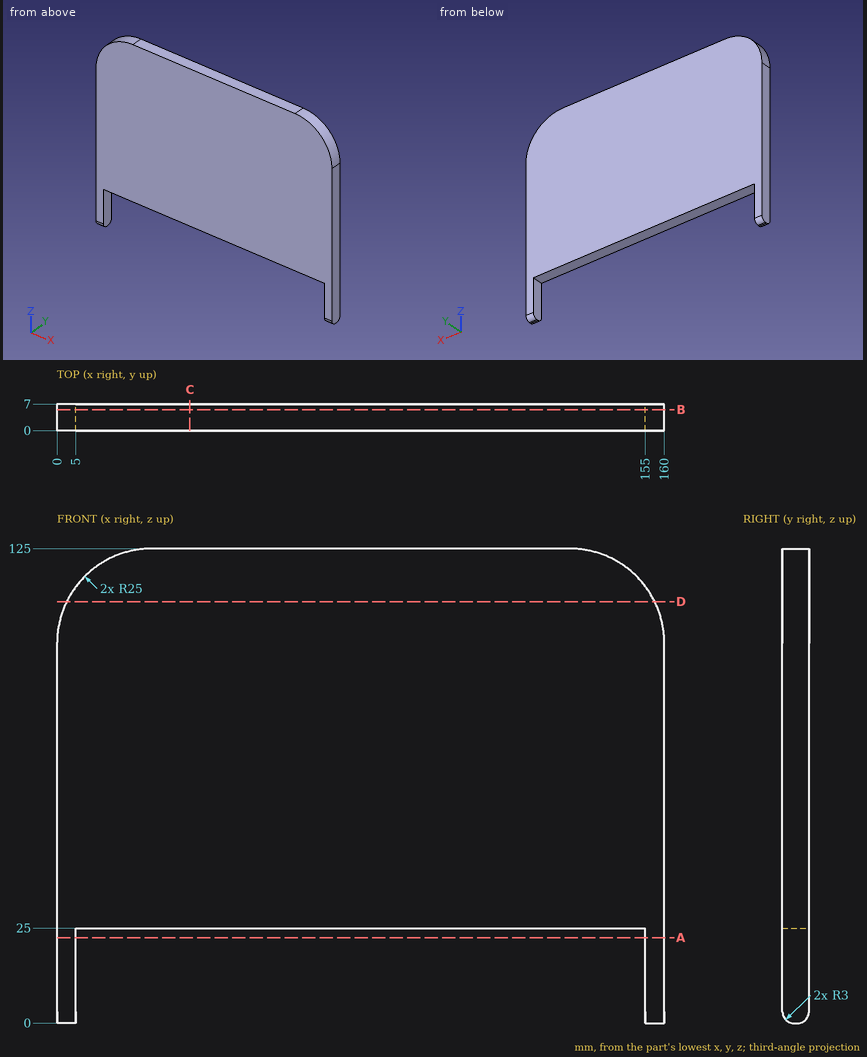
Geometry: see drawing. Coordinates: mm, zero at the bounding-box minimum. Coordinates: 2 decimals unless noted, no trailing zeros. Write each loop counter-clockwise with the first axis right and the second up, starting at its lowest first coordinate (ties: lowest second). Pieces come first, ordered by that corner, then holes. Notation, with made-up numbers: M 67,89 L 77,89 A24 ccw 77,115 Z; hole C 7.5,-13 d3. An arc over 180 degrees is marked long. Answer as a JSON object with one key per item and string values.
1. Cut plane B-B on y = 5.5. Output: boundary loops of the cut face in (x, z), plus the area to 3 significant figures.
Evaluation:
{"outline": "M 0,0.4 L 5,0.4 L 5,25 L 155,25 L 155,0.4 L 160,0.4 L 160,100 A25 ccw 135,125 L 25,125 A25 ccw 0,100 Z", "area": "16,000 mm^2"}
2. Cut plane D-D on z = 111. Output: boundary loops of the cut face in (x, y), plus the area to 3 significant figures.
Evaluation:
{"outline": "M 2.55,0 L 157.45,0 L 157.45,7 L 2.55,7 Z", "area": "1,080 mm^2"}
3. Contact query for a flat-ended pin moving along its axis: P1, Ø2, axis at x = 61.5, y = 3, coming from the -Z side. Output: stop coordinate, or through.
Evaluation:
{"P1": "z = 25"}
4. Ray query, L1, parallel to X at y = 1, z = 24.5; L2, parallel to Z at x = 41, y = 1.5; L3, parallel to Z at x = 7.5, y = 6.75. Return the intervals inside material, ascending.
Evaluation:
{"L1": "0 to 5, 155 to 160", "L2": "25 to 125", "L3": "25 to 117.85"}
5. Cut plane C-C on x = 35. Output: boundary loops of the cut face in (y, z).
Evaluation:
{"outline": "M 0,25 L 7,25 L 7,125 L 0,125 Z"}
6. Cut plane A-A on z = 22.5. Output: boundary loops of the cut face in (x, y).
Evaluation:
{"outline": "M 0,0 L 5,0 L 5,7 L 0,7 Z; M 155,0 L 160,0 L 160,7 L 155,7 Z"}
